Autodesk Inventor part; units mm, degrees
ref_plane "YZ Plane" through (0, 0, 0) normal (1, 0, 0) x (0, 1, 0)
ref_plane "XZ Plane" through (0, 0, 0) normal (0, 1, 0) x (-1, 0, 0)
ref_plane "XY Plane" through (0, 0, 0) normal (0, 0, 1) x (1, 0, 0)
sketch "Sketch1" plane through (0, 0, 0) normal (0, 0, 1) x (1, 0, 0)
  line L0 (-15, -17.5) -> (15, -17.5)
  line L1 (15, -17.5) -> (15, 17.5)
  line L2 (15, 17.5) -> (-15, 17.5)
  line L3 (-15, 17.5) -> (-15, -17.5)
  line L4 (-15, -17.5) -> (15, 17.5) construction
  line L5 (15, -17.5) -> (-15, 17.5) construction
  line L6 (-15, 17.5) -> (15, 20.1247)
  line L7 (15, 20.1247) -> (15, 17.5)
  point P0 (0, 0)
  dimension "d0" = 5
  dimension "d1" = 30
  dimension "d3" = 35
extrude "Extrusion1" add sketch "Sketch1" along normal mid plane 30
sketch "Sketch2" plane through (-15, -17.5, -15) normal (0, -1, 0) x (1, 0, 0)
  line L0 (7.5, 7.5) -> (22.5, 7.5)
  line L1 (22.5, 7.5) -> (22.5, 22.5)
  line L2 (22.5, 22.5) -> (7.5, 22.5)
  line L3 (7.5, 22.5) -> (7.5, 7.5)
  line L4 (7.5, 7.5) -> (22.5, 22.5) construction
  line L5 (22.5, 7.5) -> (7.5, 22.5) construction
  line L6 (0, 30) -> (0, 0)
  line L7 (30, 0) -> (0, 0)
  line L8 (12.5, 3) -> (17.5, 3)
  line L9 (17.5, 3) -> (17.5, 6.2)
  line L10 (17.5, 6.2) -> (12.5, 6.2)
  line L11 (12.5, 6.2) -> (12.5, 3)
  line L12 (12.5, 3) -> (17.5, 6.2) construction
  line L13 (17.5, 3) -> (12.5, 6.2) construction
  line L14 (3, 17.5) -> (6.2, 17.5)
  line L15 (6.2, 17.5) -> (6.2, 12.5)
  line L16 (6.2, 12.5) -> (3, 12.5)
  line L17 (3, 12.5) -> (3, 17.5)
  line L18 (3, 17.5) -> (6.2, 12.5) construction
  line L19 (6.2, 17.5) -> (3, 12.5) construction
  line L20 (15, 7.5) -> (15, 22.5)
  line L21 (7.5, 15) -> (22.5, 15)
  line L22 (12.5, 27) -> (17.5, 27)
  line L23 (17.5, 27) -> (17.5, 23.8)
  line L24 (17.5, 23.8) -> (12.5, 23.8)
  line L25 (12.5, 23.8) -> (12.5, 27)
  line L26 (12.5, 27) -> (17.5, 23.8) construction
  line L27 (17.5, 27) -> (12.5, 23.8) construction
  line L28 (27, 17.5) -> (23.8, 17.5)
  line L29 (23.8, 17.5) -> (23.8, 12.5)
  line L30 (23.8, 12.5) -> (27, 12.5)
  line L31 (27, 12.5) -> (27, 17.5)
  line L32 (27, 17.5) -> (23.8, 12.5) construction
  line L33 (23.8, 17.5) -> (27, 12.5) construction
  point P0 (15, 15)
  point P1 (15, 15)
  point P2 (0, 15)
  point P3 (15, 0)
  point P4 (15, 4.6)
  point P5 (4.6, 15)
  point P6 (0, 15)
  point P7 (3, 15)
  point P8 (15, 0)
  point P9 (15, 25.4)
  point P10 (25.4, 15)
  point P11 (27, 15)
  dimension "d6" = 15
  dimension "d7" = 5
  dimension "d8" = 3.2
  dimension "d9" = 3
  dimension "d10" = 3
extrude "Extrusion2" cut sketch "Sketch2" against normal through all
sketch "Sketch3" plane through (0, 0, 0) normal (0, 0, 1) x (1, 0, 0)
  line L0 (-15, -17.5) -> (-15, 17.5)
  line L1 (-15, 6.458) -> (-57.8739, 2.707)
  line L2 (-57.8739, 2.707) -> (-58.8326, 13.6651)
  line L3 (-58.8326, 13.6651) -> (-54.8478, 14.0138)
  line L4 (-54.8478, 14.0138) -> (-54.3249, 8.0366)
  line L5 (-54.3249, 8.0366) -> (-15, 11.4771)
  line L6 (15, 20.1247) -> (-15, 17.5)
  line L7 (-54.8478, 14.0138) -> (-15, 17.5)
  point P0 (0, 0)
  dimension "d14" = 4
  dimension "d15" = 5
  dimension "d16" = 6
  dimension "d17" = 40
extrude "Extrusion3" add sketch "Sketch3" along normal mid plane 20 contours L1 L2 L3 L4 L5 L0
sketch "Sketch4" plane through (-54.3249, 8.0366, 10) normal (-0.0872, 0.9962, 0) x (0.9962, 0.0872, 0)
  circle A0 centre (24, 10) radius 1.6
  line L0 (39.4751, 20) -> (39.4751, 0)
  line L1 (0, 0) -> (0, 20)
  point P0 (53.4177, 10)
  point P1 (39.4751, 10)
  dimension "d20" = 3.2
  dimension "d21" = 24
extrude "Extrusion4" cut sketch "Sketch4" against normal blind 20
sketch "Sketch5" plane through (-15, -17.5, 15) normal (-1, 0, 0) x (0, 0, 1)
  line L0 (-22.5, 36.9771) -> (-7.5, 36.9771)
  line L1 (-7.5, 36.9771) -> (-7.5, 28.9771)
  line L2 (-7.5, 28.9771) -> (-22.5, 28.9771)
  line L3 (-22.5, 28.9771) -> (-22.5, 36.9771)
  line L4 (-22.5, 36.9771) -> (-7.5, 28.9771) construction
  line L5 (-7.5, 36.9771) -> (-22.5, 28.9771) construction
  line L6 (-30, 35) -> (0, 35)
  line L7 (-25, 28.9771) -> (-5, 28.9771)
  point P0 (-15, 17.5)
  point P1 (-15, 32.9771)
  point P2 (-15, 35)
  point P3 (-15, 28.9771)
  dimension "d24" = 15
  dimension "d25" = 8
extrude "Extrusion5" cut sketch "Sketch5" against normal up to surface (22.5 mm away)
sketch "Sketch7" plane through (0, 0, 15) normal (0, 0, 1) x (1, 0, 0)
  line L0 (15, 20.1247) -> (-15, 17.5)
  line L1 (-5.9772, 18.2894) -> (5.9772, 19.3353)
  line L2 (5.9772, 19.3353) -> (6.3258, 15.3505)
  line L3 (6.3258, 15.3505) -> (-5.6285, 14.3046)
  line L4 (-5.6285, 14.3046) -> (-5.9772, 18.2894)
  line L5 (-5.9772, 18.2894) -> (6.3258, 15.3505) construction
  line L6 (5.9772, 19.3353) -> (-5.6285, 14.3046) construction
  point P0 (0, 0)
  point P1 (0, 18.8123)
  point P2 (0.1743, 16.8199)
  point P3 (0, 18.8123)
  point P4 (-5.9772, 18.2894)
  dimension "d30" = 12
  dimension "d31" = 4
extrude "Extrusion6" add sketch "Sketch7" along normal blind 8
sketch "Sketch8" plane through (15, 20.1247, 15) normal (-0.0872, 0.9962, 0) x (0.9962, 0.0872, 0)
  circle A0 centre (-15.0573, -4) radius 1.65
  line L0 (-9.0573, 0) -> (-9.0573, -8)
  line L1 (-9.0573, -8) -> (-21.0573, -8)
  line L2 (-9.0573, 0) -> (-21.0573, 0)
  point P0 (-16.6969, 15)
  point P1 (-9.0573, -4)
  point P2 (-15.0573, -8)
  point P3 (-15.0573, 0)
  dimension "d34" = 3.3
  dimension "d37" = 4
extrude "Extrusion7" cut sketch "Sketch8" against normal blind 12
mirror "Mirror1" about plane through (0, 0, 0) normal (0, 0, 1) of "Extrusion6", "Extrusion7"
extrude "Extrusion8" add sketch "Sketch3" along normal blind 3 from surface at 10
mirror "Mirror2" about plane through (0, 0, 0) normal (0, 0, 1) of "Extrusion8"
equation "\"d10\" = d9"
properties part number "Upper Path Fixation"
The listing builds one solid part. Answer for the finished solid, in the listing's coordinates (mm). A direction names the side the tool comes from. Coordinates: 2 decimals unless noted, no trailing zeros. Write each loop counter-clockwise with the first axis right and the second up, starting at its lowest first coordinate (ties: lowest second). Pieces come first, ordered by that corner, then holes. Notation, with made-up numbers: (4, -15) - (36, -15) arc R8 ccw to (36, -4) - close; hole circle Ø1 at (21.5, -33). An arc over 180 degrees is marked (long way). Return JSON: item names as keys, results as strings.
1. For a pull along X with two mould halves and no side action, classify faces 6 (the face through (-5.805, 16.325, -18.944)), 7 (the face through (0, 17, 23)), 8 (the face through (1.06, 16.93, 17.61)) as +X half, -X half, draft (parallel to the pull), parting line (faces both ways), or undercut.
Final values:
{"face 6": "-X half", "face 7": "draft", "face 8": "undercut"}
2. Each of these flat-tipped pins is pushed along its axis until it touches: pin 1 Ø7 at (x, y) = (-3.5, 5.5) entering from -Z; pin 2 Ø3 at (x, z) = (-50, 6) entering from -Y; pin 3 Ø6 at (y, z) = (-0.5, -15.5) entering from -X. Where does it stop, or does it pass through?
Final values:
{"pin 1": "z = -15", "pin 2": "y = 3.26", "pin 3": "x = -15"}
3. The part is cut by section B-B on y = -10. Determine the outline of the cut face in (x, z), then the cut area to 3 significant figures.
Final values:
{"outline": "(-15, -15) - (15, -15) - (15, 15) - (-15, 15) - close; hole (-12, -2.5) - (-8.8, -2.5) - (-8.8, 2.5) - (-12, 2.5) - close; hole (-7.5, -7.5) - (7.5, -7.5) - (7.5, 7.5) - (-7.5, 7.5) - close; hole (-2.5, -12) - (2.5, -12) - (2.5, -8.8) - (-2.5, -8.8) - close; hole (-2.5, 8.8) - (2.5, 8.8) - (2.5, 12) - (-2.5, 12) - close; hole (8.8, -2.5) - (12, -2.5) - (12, 2.5) - (8.8, 2.5) - close", "area": "611 mm^2"}
4. The part is cut by section D-D on y = 3.5. Determine the outline of the cut face in (x, z), then the cut area to 3 significant figures.
Final values:
{"outline": "(-57.94, -13) - (-48.81, -13) - (-48.81, 13) - (-57.94, 13) - close; (-15, -15) - (15, -15) - (15, 15) - (-15, 15) - close; hole (-12, -2.5) - (-8.8, -2.5) - (-8.8, 2.5) - (-12, 2.5) - close; hole (-7.5, -7.5) - (7.5, -7.5) - (7.5, 7.5) - (-7.5, 7.5) - close; hole (-2.5, -12) - (2.5, -12) - (2.5, -8.8) - (-2.5, -8.8) - close; hole (-2.5, 8.8) - (2.5, 8.8) - (2.5, 12) - (-2.5, 12) - close; hole (8.8, -2.5) - (12, -2.5) - (12, 2.5) - (8.8, 2.5) - close", "area": "848 mm^2"}
5. Consider line 1 along Z through (x, y) = (6, -1); line 2 along X through (y, z) = (-12, -9); line 3 along X through (y, z) = (-1, 0). Determine where each line is inside the solid, lowest interval first.
Final values:
{"line 1": "-15 to -7.5, 7.5 to 15", "line 2": "-15 to -2.5, 2.5 to 15", "line 3": "-15 to -12, -8.8 to -7.5, 7.5 to 8.8, 12 to 15"}
6. The part is cut by section C-C on x = 5. Determine the outline of the cut face in (y, z), then the cut area to 3 significant figures.
Final values:
{"outline": "(-17.5, -15) - (15.23, -15) - (15.23, -23) - (19.25, -23) - (19.25, -7.5) - (-17.5, -7.5) - close; (-17.5, 7.5) - (19.25, 7.5) - (19.25, 23) - (15.23, 23) - (15.23, 15) - (-17.5, 15) - close", "area": "615 mm^2"}
7. Which of the six approach directions +Z, -Z, +X, -X, +Y, -Y give full straight-line access (tool end or side, diameter ignored) to faces 1 (the face through (-37, 10, 13)), 2 (the face through (0, 1, -8.8)), 3 (the face through (-35, 13, 10)), 4 (the face through (-36.14, 4.61, -0.18)), 5 (the face through (6.154, 17.315, -18.944))?
Final values:
{"face 1": "+Z, -X, +Y, -Y", "face 2": "+Y, -Y", "face 3": "+Y", "face 4": "+Z, -Z, -Y", "face 5": "-Z, +X, +Y"}
8. The part is cut by section A-A on z = 3.5. Determine the outline of the cut face in (x, y).
Final values:
{"outline": "(-58.83, 13.67) - (-57.87, 2.71) - (-15, 6.46) - (-15, -17.5) - (-7.5, -17.5) - (-7.5, 11.48) - (-15, 11.48) - (-54.32, 8.04) - (-54.85, 14.01) - close; (7.5, -17.5) - (15, -17.5) - (15, 20.12) - (7.5, 19.47) - close"}
